from build123d import *

# Parameters (mm, degrees)
SKETCH1_R           = 10
BOSS_EXTRUDE1_DEPTH = 3
SKETCH2_W           = 5
SKETCH2_H           = 20
BOSS_EXTRUDE2_DEPTH = 3
SKETCH3_W           = 3
SKETCH3_H           = 3
BOSS_EXTRUDE3_DEPTH = 4
SKETCH4_R           = 6
CUT_EXTRUDE1_DEPTH  = 3
FILLET1_R           = 5


with BuildPart() as part:
    # Sketch1 → Boss-Extrude1 (new body)
    with BuildSketch(Plane(origin=(0, 0, 0), x_dir=(1, 0, 0), z_dir=(0, 1, 0))):
        with Locations(Location((0, 0, 0), (0, 0, 270))):
            Circle(SKETCH1_R)
    extrude(amount=BOSS_EXTRUDE1_DEPTH)

    # Sketch2 → Boss-Extrude2 (add)
    with BuildSketch(Plane(origin=(0, 3, 0), x_dir=(1, 0, 0), z_dir=(0, 1, 0))):
        with Locations((0, 19)):
            Rectangle(SKETCH2_W, SKETCH2_H)
    extrude(amount=-BOSS_EXTRUDE2_DEPTH)

    # Sketch3 → Boss-Extrude3 (add)
    with BuildSketch(Plane.ZY.offset(2.5)):
        with Locations((-27.5, 1.5)):
            Rectangle(SKETCH3_W, SKETCH3_H)
        with Locations((-21.5, 1.5)):
            Rectangle(SKETCH3_W, SKETCH3_H)
    extrude(amount=BOSS_EXTRUDE3_DEPTH)

    # Sketch4 → Cut-Extrude1 (cut)
    with BuildSketch(Plane(origin=(0, 3, 0), x_dir=(1, 0, 0), z_dir=(0, 1, 0))):
        with Locations(Location((0, 0, 0), (0, 0, 270))):
            Circle(SKETCH4_R)
    extrude(amount=-CUT_EXTRUDE1_DEPTH, mode=Mode.SUBTRACT)

    # Fillet1
    fillet1_edges = [part.edges().sort_by_distance(p)[0] for p in [
        (-2.5, 1.5, -9.682458366),
        (2.5, 1.5, -9.682458366),
    ]]
    fillet(fillet1_edges, radius=FILLET1_R)


solid = part.part
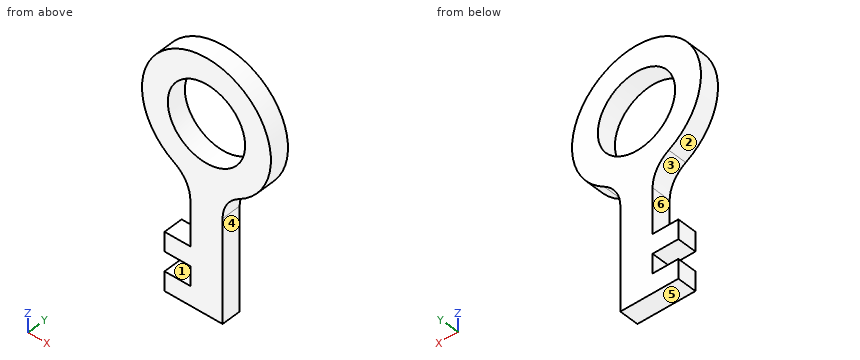
Can you work these out from the model? Positions are in its coordinate system, mm. Face numbers are marked on the shaded views. A direction names the side the tool comes from. Coordinates: 2 decimals unless noted, no trailing zeros. Order: outer loops, then holes, each group sorted by start corner. A loop starts at its lowest first (then second) coordinate and runs counter-clockwise, first axis right, second up. Notation, with made-up numbers: (23, -23) - (46, -23) arc R36 ccw to (46, 11) - close; hole circle Ø8 at (-16.75, 10). An arc over 180 degrees is marked (long way). Answer as a JSON object with one key per item and string values. Group by question number.
Q1. I need wall thicknesses on line 1 (Z direction, x = -4, y = 0.35); line 2 (X direction, y = 2.6, z = -24.5); line 3 (Z direction, x = -0.75, y = 1.8). Which ranges of each line are inside material? Lowest first, please. Write a range as from..to.
Q2. Imagine slicing it at D-D (y = 1.2). Please give me the cut outline in (x, z).
Q3. We'd pull the mould along Z, two halves only. Please class the marked faces 3, 4, 5 and 6: +Z half, -Z half, draft (parallel to the pull), parting line (faces both ways), or undercut.
Q4. Will these pins go through, and if not, where does the flat tip stop? P1, Ø0.9, axis at x = -4.5, y = 1.5, coming from the +Z side; P2, Ø1, axis at y = 0.5, z = -8, coming from the -X side; P3, Ø0.9, axis at y = 1, z = -24, coming from the +X side.
Q5. Imagine slicing it at B-B (x = 0). Please give me the cut outline in (y, z), and give its area (3 significant figures).
Q6. Imagine slicing it at C-C (x = -3.75). Please give me the cut outline in (y, z).
Q7. On a 3-axis mill with a long thin cutter (end or side, diameter ignored), from which of +Z, -Z, +X, -X, +Y, -Y can I reach the whole of each face in a straight line? I mean the marked faces 1 and 2. Say none if no direction works.
Q8. Imagine slicing it at A-A (z = 0). Please give me the cut outline in (x, y), and give its area (3 significant figures).
Determined:
{
 "1": {"line 1": "z = -29..-26, -23..-20, -9.42..-4.47, 4.47..9.17", "line 2": "x = -2.5..2.5", "line 3": "z = -29..-5.95, 5.95..9.97"},
 "2": {"outline": "(-6.5, -29) - (2.5, -29) - (2.5, -12.99) arc R5 cw to (5, -8.66) arc R10 ccw (long way) to (-5, -8.66) arc R5 cw to (-2.5, -12.99) - (-2.5, -20) - (-6.5, -20) - (-6.5, -23) - (-2.5, -23) - (-2.5, -26) - (-6.5, -26) - close; hole circle Ø12 at (0, 0)"},
 "3": {"face 3": "undercut", "face 4": "draft", "face 5": "-Z half", "face 6": "undercut"},
 "4": {"P1": "stops at z = 9.14", "P2": "stops at x = -6.61", "P3": "stops at x = 2.5"},
 "5": {"outline": "(0, -29) - (3, -29) - (3, -6) - (0, -6) - close; (0, 6) - (3, 6) - (3, 10) - (0, 10) - close", "area": "81.0 mm2"},
 "6": {"outline": "(0, -29) - (3, -29) - (3, -26) - (0, -26) - close; (0, -23) - (3, -23) - (3, -20) - (0, -20) - close; (0, -9.68) - (3, -9.68) - (3, -4.68) - (0, -4.68) - close; (0, 4.68) - (3, 4.68) - (3, 9.27) - (0, 9.27) - close"},
 "7": {"face 1": "-X, +Y, -Y", "face 2": "+Y, -Y"},
 "8": {"outline": "(-10, 0) - (-6, 0) - (-6, 3) - (-10, 3) - close; (6, 0) - (10, 0) - (10, 3) - (6, 3) - close", "area": "24.0 mm2"}
}
